from build123d import *

# Parameters (mm, degrees)
BOSS_EXTRUDE1_DEPTH            = 10
FILLET1_R                      = 5
SKETCH4_W                      = 10
SKETCH4_H                      = 8
BOSS_EXTRUDE2_DEPTH            = 5
CUT_EXTRUDE1_REACH             = 42.939
SKETCH5_R                      = 2.5
CUT_EXTRUDE1_DIRECTION_2_DEPTH = 41.938978981
SKETCH6_W                      = 10
SKETCH6_H                      = 8
BOSS_EXTRUDE3_DEPTH            = 5
SKETCH7_R                      = 2.5
CUT_EXTRUDE2_DEPTH             = 5


with BuildPart() as part:
    # Sketch1 → Boss-Extrude1 (new, symmetric)
    with BuildSketch(Plane(origin=(0, 0, 0), x_dir=(1, 0, 0), z_dir=(0, 1, 0))):
        Polygon((30, -9), (30, -13), (0, -13), (0, 0), (0, 13), (30, 13), (30, 9), (29.572320394, 9), (4, 9), (4, 0), (4, -9), (29.572320394, -9), align=None)
    extrude(amount=BOSS_EXTRUDE1_DEPTH, both=True)

    # Fillet1
    fillet1_edges = [part.edges().sort_by_distance(p)[0] for p in [
        (30, -10, -11),
        (30, -10, 11),
        (30, 10, -11),
        (30, 10, 11),
    ]]
    fillet(fillet1_edges, radius=FILLET1_R)

    # Sketch4 → Boss-Extrude2 (add)
    with BuildSketch(Plane.XY.offset(13)):
        with Locations((10, 0)):
            Rectangle(SKETCH4_W, SKETCH4_H)
    extrude(amount=BOSS_EXTRUDE2_DEPTH)

    # Cut-Extrude1: up to this face of the body (flat: up to its plane)
    cut_extrude1_end = Plane(part.part.faces().sort_by_distance((14.747199742, 0, -13))[0])
    # Sketch5 → Cut-Extrude1 (cut, up to the picked face)
    with BuildSketch(Plane.XY.offset(13), mode=Mode.PRIVATE) as cut_extrude1_sk1:
        with Locations(Location((23, 0, 0), (0, 0, 180))):
            Circle(SKETCH5_R)
    cut_extrude1_tool1 = split(extrude(cut_extrude1_sk1.sketch, amount=-CUT_EXTRUDE1_REACH, mode=Mode.PRIVATE), bisect_by=cut_extrude1_end, keep=Keep.BOTH, mode=Mode.PRIVATE)
    add(cut_extrude1_tool1.solids().sort_by(Axis((23, 0, 13), (0, 0, -1)))[0], mode=Mode.SUBTRACT)

    # Sketch5 → Cut-Extrude1 direction 2 (cut)
    with BuildSketch(Plane.XY.offset(13)):
        with Locations(Location((23, 0, 0), (0, 0, 180))):
            Circle(SKETCH5_R)
    extrude(amount=CUT_EXTRUDE1_DIRECTION_2_DEPTH, mode=Mode.SUBTRACT)

    # Sketch6 → Boss-Extrude3 (add)
    with BuildSketch(Plane(origin=(0, 0, -13), x_dir=(-1, 0, 0), z_dir=(0, 0, -1))):
        with Locations((-10, 0)):
            Rectangle(SKETCH6_W, SKETCH6_H)
    extrude(amount=BOSS_EXTRUDE3_DEPTH)

    # Sketch7 → Cut-Extrude2 (cut)
    with BuildSketch(Plane.ZY):
        Circle(SKETCH7_R)
    extrude(amount=-CUT_EXTRUDE2_DEPTH, mode=Mode.SUBTRACT)


solid = part.part
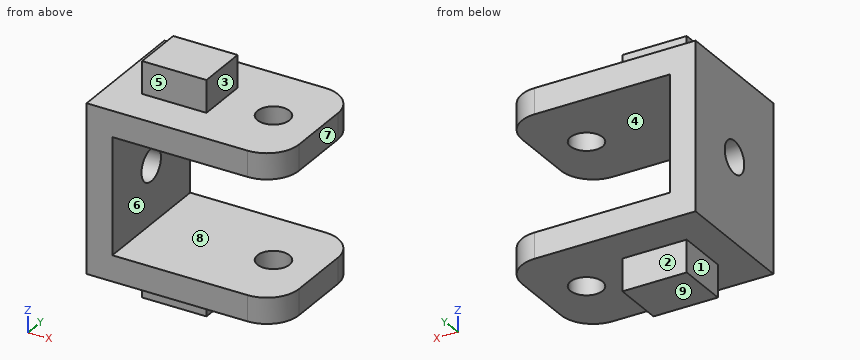
Source: CAD feature listing. Evaluate the final solid. Frame: model axes, mm. Face numbers are marked on the shaded views. A direction names the side the tool comes from. Give positions to 0.01 mm unless a question says otherwise; leave off trailing zeros. Order: outer loops, then holes, each group sorted by start corner. A loop starts at its lowest first (then second) coordinate and runs counter-clockwise, first axis right, second up. Notation, with made-up numbers: (15, 44.5) -> (57, 44.5) arc R34 cw to (57, 75.5) -> close; hole circle Ø11 at (-22, -28). An arc over 180 degrees is marked (long way). Use a Markdown table: item, result.
1) Section query A-A, the plane y = 0. Return the cut outline in (x, z).
Answer list:
| item | result |
|---|---|
| outline | (0, -13) -> (5, -13) -> (5, -18) -> (15, -18) -> (15, -13) -> (20.5, -13) -> (20.5, -9) -> (4, -9) -> (4, -2.5) -> (0, -2.5) -> close; (0, 2.5) -> (4, 2.5) -> (4, 9) -> (20.5, 9) -> (20.5, 13) -> (15, 13) -> (15, 18) -> (5, 18) -> (5, 13) -> (0, 13) -> close; (25.5, -13) -> (30, -13) -> (30, -9) -> (25.5, -9) -> close; (25.5, 9) -> (30, 9) -> (30, 13) -> (25.5, 13) -> close |
2) Section query D-D, the plane x = 14.25. Return the cut outline in (y, z), then the cut area to 3 significant figures.
Answer list:
| item | result |
|---|---|
| outline | (-10, -13) -> (-4, -13) -> (-4, -18) -> (4, -18) -> (4, -13) -> (10, -13) -> (10, -9) -> (-10, -9) -> close; (-10, 9) -> (10, 9) -> (10, 13) -> (4, 13) -> (4, 18) -> (-4, 18) -> (-4, 13) -> (-10, 13) -> close |
| area | 240 mm² |
3) Section query C-C, the plane x = 23. Return the cut outline in (y, z).
Answer list:
| item | result |
|---|---|
| outline | (-10, -13) -> (-2.5, -13) -> (-2.5, -9) -> (-10, -9) -> close; (-10, 9) -> (-2.5, 9) -> (-2.5, 13) -> (-10, 13) -> close; (2.5, -13) -> (10, -13) -> (10, -9) -> (2.5, -9) -> close; (2.5, 9) -> (10, 9) -> (10, 13) -> (2.5, 13) -> close |
4) Section query B-B, the plane z = 0. Return the cut outline in (x, y).
Answer list:
| item | result |
|---|---|
| outline | (0, -10) -> (4, -10) -> (4, -2.5) -> (0, -2.5) -> close; (0, 2.5) -> (4, 2.5) -> (4, 10) -> (0, 10) -> close |
5) Reachability of the marked faces 1, 2, 3, 4 and 5 from +Z, -Z, +X, -X, +Y, -Y: full face, straight path, thin tool, end or side. Return the list, or none.
Answer list:
| item | result |
|---|---|
| face 1 | -Z, -X, +Y, -Y |
| face 2 | -Z, +X, -X, +Y |
| face 3 | +Z, +X, +Y, -Y |
| face 4 | +X, +Y, -Y |
| face 5 | +Z, +X, -X, -Y |
6) Mould query, pull axis Z, two halves, no side actions, for the marked faces 6, 7, 8 and 9. Classes: +Z half, -Z half, draft (parallel to the pull), parting line (faces both ways), or undercut.
Answer list:
| item | result |
|---|---|
| face 6 | undercut |
| face 7 | draft |
| face 8 | undercut |
| face 9 | -Z half |
7) Contact query for flat-ended pins moving along their axis: P1, Ø2, axis at x = 8, y = 6.5, coming from the -Z side; P2, Ø1.5, axis at x = 9.5, z = -16, coming from the +Y side; P3, Ø3, axis at x = 19.5, y = -0.5, coming from the +Z side; P4, Ø1.5, axis at x = 13, z = -7.5, coming from the +Y side. Output: stop coordinate, or through.
Answer list:
| item | result |
|---|---|
| P1 | z = -13 |
| P2 | y = 4 |
| P3 | z = 13 |
| P4 | through |
8) Ray query, line 1 along Y through (x, z) = (23, -11.3); line 2 along Z through (x, y) = (12.25, -1.5); line 3 along Z through (x, y) = (5.75, -9). Return the intervals inside material, ascending. Write a range as [from, to].
Answer list:
| item | result |
|---|---|
| line 1 | [-10, -2.5], [2.5, 10] |
| line 2 | [-18, -9], [9, 18] |
| line 3 | [-13, -9], [9, 13] |
